```python
from build123d import *

# Parameters (mm, degrees)
F0_R          = 25.4
F0_R_2        = 12.7
F1_DEPTH      = 76.2
F3_DEPTH      = 12.7
F5_START      = -12.7
F5_DEPTH      = 12.7
F7_DEPTH      = 25.4
F7_DEPTH_BACK = 12.7
F9_DEPTH      = 38.1
F10_W         = 25.4
F10_H         = 12.7
F11_DEPTH     = 25.4


with BuildPart() as f1:
    # F0 (on Front) → F1 (new body)
    with BuildSketch(Plane.XZ):
        Circle(F0_R)
        Circle(F0_R_2, mode=Mode.SUBTRACT)
    extrude(amount=-F1_DEPTH)

    # F2 (on face) → F3 (cut)
    with BuildSketch(Plane.XZ):
        with BuildLine():
            Line((8.1350766981, 9.7524626181), (23.4531335408, 9.7524626181))
            ThreePointArc((23.4531335408, 9.7524626181), (0, 25.4), (-23.4531335408, 9.7524626181))
            Line((-23.4531335408, 9.7524626181), (-8.1350766981, 9.7524626181))
            ThreePointArc((-8.1350766981, 9.7524626181), (0, 12.7), (8.1350766981, 9.7524626181))
        make_face()
    extrude(amount=-F3_DEPTH, mode=Mode.SUBTRACT)

    # F4 (on face) → F5 (cut)
    with BuildSketch(Plane.XZ.offset(F5_START)):
        with BuildLine():
            Line((23.5464301965, -9.525), (38.1, -9.525))
            Line((38.1, -9.525), (38.1, 25.4))
            Line((38.1, 25.4), (-38.1, 25.4))
            Line((-38.1, 25.4), (-38.1, -9.525))
            Line((-38.1, -9.525), (-23.5464301965, -9.525))
            ThreePointArc((-23.5464301965, -9.525), (-25.39970254, 0.1229263078), (-23.4531335408, 9.7524626181))
            Line((-23.4531335408, 9.7524626181), (-8.1350766981, 9.7524626181))
            ThreePointArc((-8.1350766981, 9.7524626181), (-12.698798549, 0.1746866087), (-8.4002604126, -9.525))
            Line((-8.4002604126, -9.525), (8.4002604126, -9.525))
            ThreePointArc((8.4002604126, -9.525), (11.5752604126, -5.2252604126), (12.7, 0))
            ThreePointArc((12.7, 0), (11.5022926859, 5.3839820735), (8.1350766981, 9.7524626181))
            Line((8.1350766981, 9.7524626181), (23.4531335408, 9.7524626181))
            ThreePointArc((23.4531335408, 9.7524626181), (24.908528579, 4.9724444724), (25.4, 0))
            ThreePointArc((25.4, 0), (24.9323016085, -4.8518384664), (23.5464301965, -9.525))
        make_face()
        with BuildLine():
            ThreePointArc((-23.4531335408, 9.7524626181), (-25.39970254, 0.1229263078), (-23.5464301965, -9.525))
            Line((-23.5464301965, -9.525), (-8.4002604126, -9.525))
            ThreePointArc((-8.4002604126, -9.525), (-12.698798549, 0.1746866087), (-8.1350766981, 9.7524626181))
            Line((-8.1350766981, 9.7524626181), (-23.4531335408, 9.7524626181))
        make_face()
        with BuildLine():
            Line((8.4002604126, -9.525), (23.5464301965, -9.525))
            ThreePointArc((23.5464301965, -9.525), (24.9323016085, -4.8518384664), (25.4, 0))
            ThreePointArc((25.4, 0), (24.908528579, 4.9724444724), (23.4531335408, 9.7524626181))
            Line((23.4531335408, 9.7524626181), (8.1350766981, 9.7524626181))
            ThreePointArc((8.1350766981, 9.7524626181), (11.5022926859, 5.3839820735), (12.7, 0))
            ThreePointArc((12.7, 0), (11.5752604126, -5.2252604126), (8.4002604126, -9.525))
        make_face()
    extrude(amount=-F5_DEPTH, mode=Mode.SUBTRACT)

    # F6 (on Right) → F7 (join, two sides)
    with BuildSketch(Plane.YZ) as f7_sk:
        Polygon((38.1, 0), (76.2, 0), (76.2, 50.8), align=None)
    extrude(amount=F7_DEPTH)
    extrude(f7_sk.sketch, amount=-F7_DEPTH_BACK)

    # F8 (on face) → F9 (cut)
    with BuildSketch(Plane(origin=(0, 76.2, 0), x_dir=(-1, 0, 0), z_dir=(0, 1, 0))):
        with BuildLine():
            Line((-12.7, 0), (12.7, 0))
            ThreePointArc((12.7, 0), (0, 12.7), (-12.7, 0))
        make_face()
    extrude(amount=-F9_DEPTH, mode=Mode.SUBTRACT)

    # F10 (on face) → F11 (cut)
    with BuildSketch(Plane(origin=(0, 76.2, 0), x_dir=(-1, 0, 0), z_dir=(0, 1, 0))):
        with Locations((0, 44.45)):
            Rectangle(F10_W, F10_H)
    extrude(amount=-F11_DEPTH, mode=Mode.SUBTRACT)


solid = f1.part
```
Model file for the job. Use its own axes, mm. A direction names the side the tool comes from. Coordinates: 2 decimals unless noted, no trailing zeros. Order: outer loops, then holes, each group sorted by start corner. A loop starts at its lowest first (then second) coordinate and runs counter-clockwise, first axis right, second up. Notation, with made-up numbers: M 20.5,-37 L 29.5,-37 A24 ccw 29.5,-3 Z; hole C -9,62 d11. An arc over 180 degrees is marked long. Answer as CSV lines item,"result".
(1) 3-axis set-ups, long thin cutter, end or side, ignore diameter. For faces 5 (the flat face through (16, 6, 9.752)), 6 (the flat face through (-12.7, 68, 28)), 7 (the flat face through (25.4, 65, 14)), 8 (the flat face through (16, 19, -9.525)), 9 (the flat face through (6, 76.2, 12)): which of +Z, -Z, +X, -X, +Y, -Y reach the whole face in a straight line?
Geometry says:
face 5,"+Z, +X, -X, -Y"
face 6,"+Z, -X, +Y, -Y"
face 7,"+Z, -Z, +X, +Y, -Y"
face 8,"+Z, +X, -X"
face 9,"+Z, -Z, +X, -X, +Y"
(2) Band-saw the part on A-A, the plane x = 0. List the corners of the cut face in (y, z) (3 decimals).
Geometry says:
outline,"M 0,-25.4 L 76.2,-25.4 L 76.2,-12.7 L 0,-12.7 Z; M 25.4,12.7 L 76.2,12.7 L 76.2,38.1 L 66.675,38.1 L 57.15,25.4 L 25.4,25.4 Z"
(3) Band-saw the part on D-D, the plane z = 26.5. List the corners of the cut face in (x, y) (3 decimals), then the cut area to 3 significant figures.
Geometry says:
outline,"M -12.7,57.975 L 25.4,57.975 L 25.4,76.2 L -12.7,76.2 Z"
area,"694 mm2"
(4) Band-saw the part on B-B, the plane z = -4. List the corners of the cut face in (x, y), then the cut area to 3 significant figures.
Geometry says:
outline,"M -25.08,0 L -12.05,0 L -12.05,12.7 L -25.08,12.7 Z; M -25.08,25.4 L -12.05,25.4 L -12.05,76.2 L -25.08,76.2 Z; M 12.05,0 L 25.08,0 L 25.08,12.7 L 12.05,12.7 Z; M 12.05,25.4 L 25.08,25.4 L 25.08,76.2 L 12.05,76.2 Z"
area,"1,650 mm2"
(5) Band-saw the part on C-C, the plane y = 17. List the corners of the cut face in (x, z) (3 decimals).
Geometry says:
outline,"M -23.546,-9.525 A25.4 ccw 23.546,-9.525 L 8.4,-9.525 A12.7 cw -8.4,-9.525 Z"
(6) Pull direction Y, two halves, no side cores. Call faces 1 (the flat face through (-16, 19, -9.525)), 2 (the flat face through (-6, 0, -11.5)), 3 (the flat face through (-16, 6, 9.752)), 4 (the flat face through (19, 12.7, 0)): +Y half, -Y half, draft (parallel to the pull), parting line (faces both ways), or undercut.
Geometry says:
face 1,"undercut"
face 2,"-Y half"
face 3,"draft"
face 4,"undercut"
(7) Flat gauge pins, fed straight in: pin 1 (14 mm diameter, centred on x = -12.5, y = 6, fed in from +Z); pin 2 (5 mm diameter, centred on x = -4.5, y = 69.5, fed in from +Z); pin 3 (5 mm diameter, centred on y = 40.5, z = -6, fed in from -X); pin 4 (12 mm diameter, centred on y = 32, z = 35.5, fed in from +X). Where does each tip first touch, or does it go through?
Geometry says:
pin 1,"stops at z = 9.75"
pin 2,"stops at z = 38.1"
pin 3,"stops at x = -25.16"
pin 4,"passes through"
(8) Wall check: line 1 along Z through (x, y) = (0, 51); line 2 along Y through (x, z) = (17, 5.5). Give the ranges that are in metal, low to high.
Geometry says:
line 1,"z = -25.4 to -12.7, 12.7 to 25.4"
line 2,"y = 0 to 12.7, 25.4 to 76.2"
